Could you check a few things on this model? Use its own coordinates, in mm. A direction names the side the tool comes from. Give positions to 0.01 mm unless a question says otherwise; leave off trailing zeros. Order: outer loops, then holes, each group sorted by start corner. A loop starts at its lowest first (then second) coordinate and runs counter-clockwise, first axis right, second up. Notation, with made-up numbers: M -32.75,54.25 L -0.75,54.25 A10 cw -0.75,64.25 Z; hole C -13.75,5 d7. An arc over 180 degrees is marked long. Use a Markdown table: item, result. Add a question column.
Item 1: Suppose I cut it at B-B on y = 1.25. Write out the boundary of the cut face in (x, z).
Item 2: For faces 1 (the face through (8, 0, 1)), 2 (the face through (-0.8, -9.6, 100)), which set-ups out of +Z, -Z, +X, -X, +Y, -Y let a thin tool reach every point of the face, with its end or its side?
Item 3: Suppose I cut it at A-A on z = -18.5. Write out the boundary of the cut face in (x, y).
Item 4: I'm going to push a flat-ended pin straight in: pin 1 Ø6 at (x, y) = (-1.5, 4.5) entering from -Z. Where does the tip first touch, or does it pass through?
Item 5: If we mould it in two halves opening along Y, with no side actions, what happens to faces 3 (the face through (-0.8, -9.6, -100)), 4 (the face through (0, -10, 1)), 5 (the face through (0, -8, 1))? For each: released by +Y, released by -Y, zero draft, split by the parting line, or undercut.
Item 6: If I drill on L1, parallel to X at y = 2.5, z = -31.5; L2, parallel to Z at x = 8.25, y = 8, over which ranges is the centre line in solid material (lowest first)? Write a range as from..to.
from build123d import *

# Parameters (mm, degrees)
F0_W     = 20
F0_H     = 20
F0_W_2   = 16
F0_H_2   = 16
F1_DEPTH = 100
F2_SIZE  = 1


with BuildPart() as f1:
    # F0 (on Top) → F1 (new body, symmetric)
    with BuildSketch(Plane.XY):
        Rectangle(F0_W, F0_H)
        Rectangle(F0_W_2, F0_H_2, mode=Mode.SUBTRACT)
    extrude(amount=F1_DEPTH, both=True)

    # F2
    f2_edges = [f1.edges().sort_by_distance(p)[0] for p in [
        (0, 8, 100),
        (-8, 0, 100),
        (8, 0, 100),
        (0, -8, 100),
        (0, 8, -100),
        (8, 0, -100),
        (0, -8, -100),
        (-8, 0, -100),
    ]]
    chamfer(f2_edges, length=F2_SIZE)


solid = f1.part
Findings below:
| question | item | result |
|---|---|---|
| 1 | outline | M -10,-100 L -9,-100 L -8,-99 L -8,99 L -9,100 L -10,100 Z; M 8,-99 L 9,-100 L 10,-100 L 10,100 L 9,100 L 8,99 Z |
| 2 | face 1 | +Z, -Z |
| 2 | face 2 | +Z, +X, -X, +Y, -Y |
| 3 | outline | M -10,-10 L 10,-10 L 10,10 L -10,10 Z; hole M -8,-8 L 8,-8 L 8,8 L -8,8 Z |
| 4 | pin 1 | passes through |
| 5 | face 3 | zero draft |
| 5 | face 4 | released by -Y |
| 5 | face 5 | undercut |
| 6 | L1 | x = -10..-8, 8..10 |
| 6 | L2 | z = -99.25..99.25 |
